Check sheet for the drawn part. Datum: minimum x, y, z corner. Units: mm. Round coordinates to 2 decimals unless told otherwise and drop trailing zeros. Write each loop counter-clockwise with the first axis right and the second up, starting at its lowest first coordinate (ties: lowest second). Pieces come first, ordered by that corner, then holes.
Item 1: Cross-section at C-C on y = 63. Enter the section's corners in (x, z).
Item 2: Material ranges on line 1 (Y direction, x = 7.5, z = 4); line 2 (Y direction, x = 3, z = 4); line 3 (X direction, y = 66, z = 5), recorded low to high.
Item 3: Cross-section at B-B on z = 1.5. Enter the section's corners in (x, y).
Item 4: Cross-section at A-A on z = 4. Enter the section's corners in (x, y), plus the area to 3 significant figures.
Item 5: Cross-section at D-D on y = 41.5. Enter the section's corners in (x, z), plus the area to 3 significant figures.
Item 6: Go/stop test with flat-tipped pins: pin 1 Ø1 at (y, z) = (38, 4.5) entering from +X; pin 2 Ø1.8 at (x, y) = (4, 66) entering from +Z; pin 3 Ø3 at (x, y) = (6, 29) entering from +Z; pin 4 Ø4 at (y, z) = (59, 1) entering from +X. Record where each tip stops, or that it passes through.
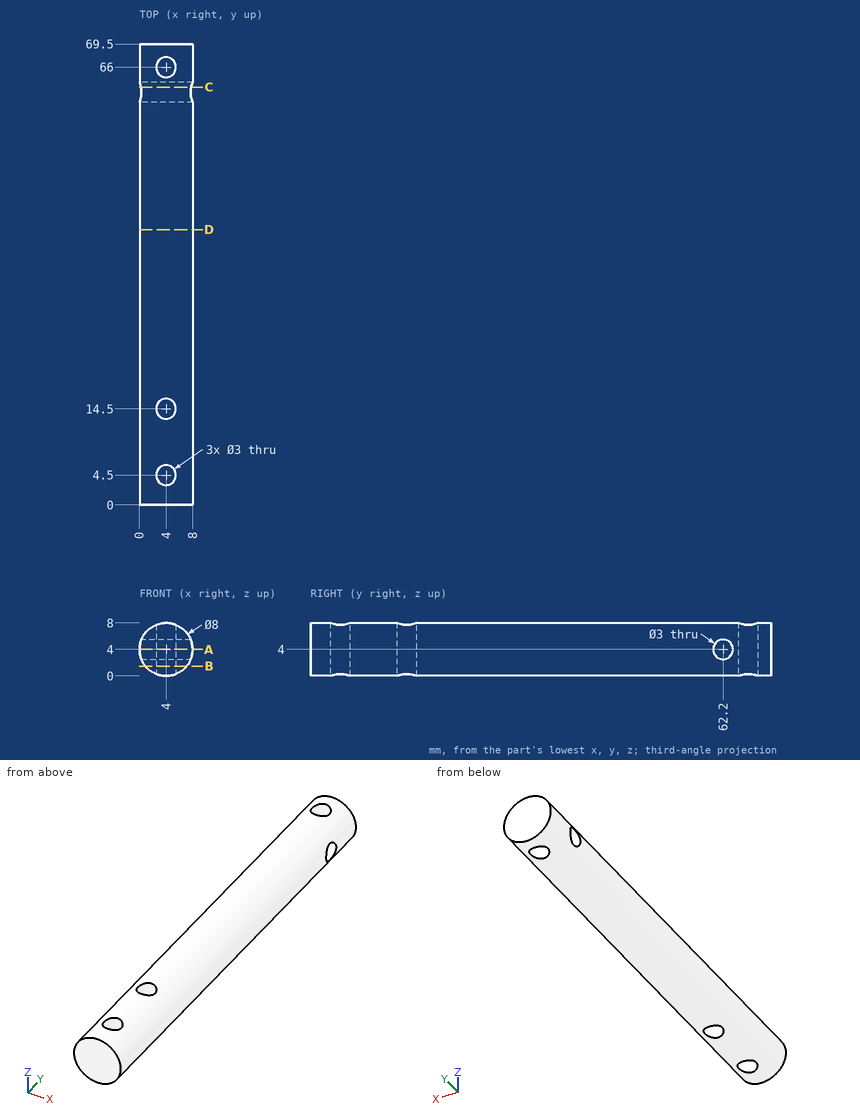
Response values:
1. outline: (0.21, 2.73) arc R4 ccw to (7.79, 2.73) - close; (0.21, 5.27) - (7.79, 5.27) arc R4 ccw to start
2. line 1: y = 0 to 60.7, 63.7 to 69.5
2. line 2: y = 0 to 3.38, 5.62 to 13.38, 15.62 to 60.7, 63.7 to 64.88, 67.12 to 69.5
2. line 3: x = 0.13 to 2.5, 5.5 to 7.87
3. outline: (0.88, 0) - (7.12, 0) - (7.12, 69.5) - (0.88, 69.5) - close; hole circle Ø3 at (4, 4.5); hole circle Ø3 at (4, 14.5); hole circle Ø3 at (4, 66)
4. outline: (0, 0) - (8, 0) - (8, 60.7) - (0, 60.7) - close; (0, 63.7) - (8, 63.7) - (8, 69.5) - (0, 69.5) - close; hole circle Ø3 at (4, 4.5); hole circle Ø3 at (4, 14.5); hole circle Ø3 at (4, 66)
4. area: 511 mm2
5. outline: circle Ø8 at (4, 4)
5. area: 50.3 mm2
6. pin 1: stops at x = 8
6. pin 2: passes through
6. pin 3: stops at z = 7.97
6. pin 4: stops at x = 7.87
